Verification items for the finished model (mm, model axes). Face numbers are marked on the shaded views. A direction names the side the tool comes from. Give positions to 0.01 mm unless a question says otherwise; leave off trailing zeros. Loops run counter-clockwise (first coordinate to the right, second up) from the corner with the lowest first, then second, coordinate; pieces in that order, holes last. Notation, with made-up numbers: (-24, 52) - (4, 52) arc R28 ccw to (4, 76) - close; hole circle Ø11 at (43.25, 36.25). An arc over 180 degrees is marked (long way). One line per item, written item: value. Start each with the question number.
1. Sectioned sample at B-B (y = 177). Record the cut outline in (x, z), plus the area to 3 significant figures.
2. Scan line: L1, parallel to Z at x = -1.75, y = 160.5. Record every from-to range of solid material in increasing order. Write a range as [from, to].
3. Sectioned sample at C-C (z = 7.25). Record the cut outline in (x, y), plus the area to 3 significant figures.
4. Gauge pin test, flat end, axial feed: pin 1 (2 mm diameter, centred on x = -5.5, z = 8.5, fed in from -Y). Record the tip position at first contact, or that the pin passes through.
5. Access from +Z, -Z, +X, -X, +Y, -Y to the whole of each face (thin tool, end or side, straight path). Record for the marked faces 1 and 2.
6. Mould release check, pull along Z, two halves, no side actions. Record for the marked faces 3, 4 and 5: pulls with the +Z half, pulls with the -Z half, needs draft (parallel to the pull), parting line crosses it, or undercut.
7. Sectioned sample at A-A (x = -8). Record the cut outline in (y, z).
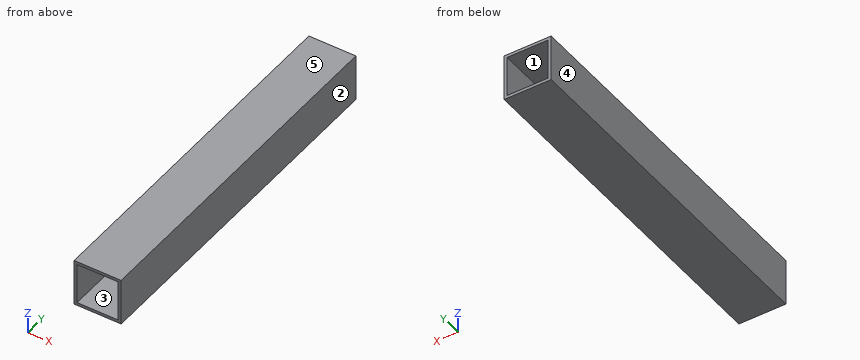
Autodesk Inventor part; units mm, degrees
ref_plane "YZ Plane" through (0, 0, 0) normal (1, 0, 0) x (0, 1, 0)
ref_plane "XZ Plane" through (0, 0, 0) normal (0, 1, 0) x (-1, 0, 0)
ref_plane "XY Plane" through (0, 0, 0) normal (0, 0, 1) x (1, 0, 0)
sketch "Sketch1" plane through (0, 0, 0) normal (0, 1, 0) x (-1, 0, 0)
  line L0 (12.7, 0) -> (12.7, -12.7)
  line L1 (12.7, -12.7) -> (0, -12.7)
  line L2 (0, 0) -> (24.2319, 0) construction
  line L3 (0, 0) -> (0, -21.2534) construction
  line L4 (12.7, 0) -> (12.7, 12.7)
  line L5 (12.7, 12.7) -> (0, 12.7)
  line L6 (-12.7, 0) -> (-12.7, -12.7)
  line L7 (-12.7, -12.7) -> (0, -12.7)
  line L8 (-12.7, 0) -> (-12.7, 12.7)
  line L9 (-12.7, 12.7) -> (0, 12.7)
  line L10 (0, -11.1125) -> (11.1125, -11.1125)
  line L11 (11.1125, -11.1125) -> (11.1125, 0)
  line L12 (11.1125, 0) -> (11.1125, 11.1125)
  line L13 (11.1125, 11.1125) -> (0, 11.1125)
  line L14 (0, 11.1125) -> (-11.1125, 11.1125)
  line L15 (-11.1125, 11.1125) -> (-11.1125, 0)
  line L16 (-11.1125, 0) -> (-11.1125, -11.1125)
  line L17 (-11.1125, -11.1125) -> (0, -11.1125)
  dimension "d1" = 12.7
  dimension "d2" = 12.7
  dimension "d3" = 12.7
  dimension "d4" = 12.7
  dimension "d5" = 24.2319
  dimension "d6" = 21.2534
  dimension "d7" = 1.5875
extrude "Extrusion1" add sketch "Sketch1" along normal blind 190.5
equation "\"d3\" = d1"
properties part number "gripper arm bracket"
Results are:
1. outline: (-12.7, -12.7) - (12.7, -12.7) - (12.7, 12.7) - (-12.7, 12.7) - close; hole (-11.11, -11.11) - (11.11, -11.11) - (11.11, 11.11) - (-11.11, 11.11) - close
1. area: 151 mm^2
2. L1: z = [-12.7, -11.11], [11.11, 12.7]
3. outline: (-12.7, 0) - (-11.11, 0) - (-11.11, 190.5) - (-12.7, 190.5) - close; (11.11, 0) - (12.7, 0) - (12.7, 190.5) - (11.11, 190.5) - close
3. area: 605 mm^2
4. pin 1: passes through
5. face 1: +Y, -Y
5. face 2: +Z, -Z, +X, +Y, -Y
6. face 3: undercut
6. face 4: needs draft
6. face 5: pulls with the +Z half
7. outline: (0, -12.7) - (190.5, -12.7) - (190.5, -11.11) - (0, -11.11) - close; (0, 11.11) - (190.5, 11.11) - (190.5, 12.7) - (0, 12.7) - close
